Work out the finished part from the listing and answer in its coordinate system (mm). Round coordinates to 2 decimals unless told otherwise and drop trailing zeros. Order: outer loops, then holes, each group sorted by start corner. A loop starts at its lowest first (then second) coordinate and runs counter-clockwise, first axis right, second up. Notation, with made-up numbers: (78.25, -34) - (87.25, -34) arc R12 cw to (87.25, -18) - close; hole circle Ø2 at (1.25, 56.5). An arc over 180 degrees is marked (long way). Answer in a Markdown table with one row per item.
from build123d import *

# Parameters (mm, degrees)
SKETCH1_R           = 1.75
SKETCH1_R_2         = 1
BOSS_EXTRUDE1_DEPTH = 2
SKETCH3_R           = 1.75
SKETCH3_W           = 40
SKETCH3_H           = 10
CUT_EXTRUDE2_DEPTH  = 10
FILLET1_R           = 2
FILLET2_R           = 5
FILLET3_R           = 10
SKETCH4_R           = 1.5
CUT_EXTRUDE3_DEPTH  = 10


with BuildPart() as part:
    # Sketch1 → Boss-Extrude1 (new body)
    with BuildSketch(Plane(origin=(0, 0, 0), x_dir=(1, 0, 0), z_dir=(0, 1, 0))):
        Polygon((-90, 32.535953793), (-90, -32.464046207), (90, -32.464046207), (90, 32.535953793), (50, 32.535953793), (50, 72.535953793), (-50, 72.535953793), (-50, 32.535953793), align=None)
        with Locations((-85, -27.535953793)):
            Circle(SKETCH1_R, mode=Mode.SUBTRACT)
        with Locations((85, -27.535953793)):
            Circle(SKETCH1_R, mode=Mode.SUBTRACT)
        with Locations((-30, -27.535953793)):
            Circle(SKETCH1_R, mode=Mode.SUBTRACT)
        with Locations((30, -27.535953793)):
            Circle(SKETCH1_R, mode=Mode.SUBTRACT)
        with Locations((-67, 17.464046207)):
            Circle(SKETCH1_R, mode=Mode.SUBTRACT)
        with Locations((67, 17.464046207)):
            Circle(SKETCH1_R, mode=Mode.SUBTRACT)
        with Locations((-47, 69.535953793)):
            Circle(SKETCH1_R_2, mode=Mode.SUBTRACT)
        with Locations((-47, 25.035953793)):
            Circle(SKETCH1_R_2, mode=Mode.SUBTRACT)
        with Locations((47, 25.035953793)):
            Circle(SKETCH1_R_2, mode=Mode.SUBTRACT)
        with Locations((47, 69.535953793)):
            Circle(SKETCH1_R_2, mode=Mode.SUBTRACT)
    extrude(amount=BOSS_EXTRUDE1_DEPTH)

    # Sketch3 → Cut-Extrude2 (cut)
    with BuildSketch(Plane(origin=(0, 2, 0), x_dir=(1, 0, 0), z_dir=(0, 1, 0))):
        with Locations((-43, 62.464046207)):
            Circle(SKETCH3_R)
        with Locations((43, 62.464046207)):
            Circle(SKETCH3_R)
        Polygon((2.5, 48.535953793), (42.5, 48.535953793), (42.5, 46.535953793), (38, 46.535953793), (38, 6.535953793), (25, 6.535953793), (25, -13.464046207), (-25, -13.464046207), (-25, 6.535953793), (-38, 6.535953793), (-38, 46.535953793), (-42.5, 46.535953793), (-42.5, 48.535953793), (-2.5, 48.535953793), (-2.5, 53.535953793), (2.5, 53.535953793), align=None)
        with Locations((70, 27.535953793)):
            Rectangle(SKETCH3_W, SKETCH3_H)
        with Locations((-70, 27.535953793)):
            Rectangle(SKETCH3_W, SKETCH3_H)
    extrude(amount=-CUT_EXTRUDE2_DEPTH, mode=Mode.SUBTRACT)

    # Fillet1
    fillet1_edges = [part.edges().sort_by_distance(p)[0] for p in [
        (-50, 1, -72.535953793),
        (50, 1, -72.535953793),
    ]]
    fillet(fillet1_edges, radius=FILLET1_R)

    # Fillet2
    fillet2_edges = [part.edges().sort_by_distance(p)[0] for p in [
        (90, 1, -22.535953793),
        (25, 1, -6.535953793),
        (-25, 1, -6.535953793),
        (90, 1, 32.464046207),
        (-90, 1, 32.464046207),
        (-90, 1, -22.535953793),
    ]]
    fillet(fillet2_edges, radius=FILLET2_R)

    # Fillet3
    fillet3_edges = [part.edges().sort_by_distance(p)[0] for p in [
        (50, 1, -22.535953793),
        (-50, 1, -22.535953793),
    ]]
    fillet(fillet3_edges, radius=FILLET3_R)

    # Sketch4 → Cut-Extrude3 (cut)
    with BuildSketch(Plane(origin=(0, 2, 0), x_dir=(1, 0, 0), z_dir=(0, 1, 0))):
        with Locations((-82, 10.535953793)):
            Circle(SKETCH4_R)
        with Locations((-82, -4.464046207)):
            Circle(SKETCH4_R)
        with Locations((82, 10.535953793)):
            Circle(SKETCH4_R)
        with Locations((82, -4.464046207)):
            Circle(SKETCH4_R)
    extrude(amount=-CUT_EXTRUDE3_DEPTH, mode=Mode.SUBTRACT)


solid = part.part
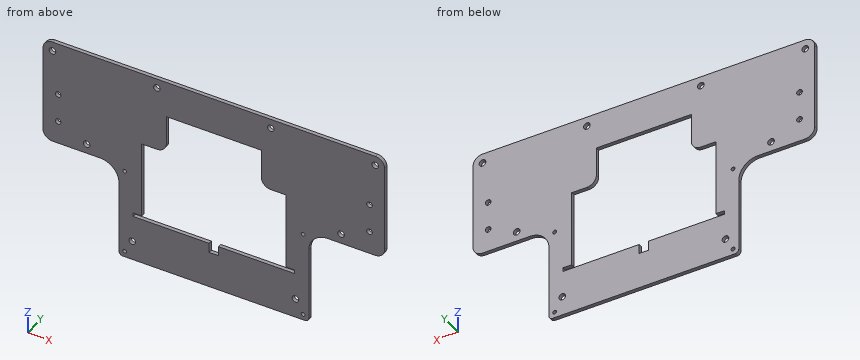
1) Find section A-A, the plane x = 18.5. Give the vertices of the cut face in (y, z).
Filled in:
| item | result |
|---|---|
| outline | (0, -72.54) - (2, -72.54) - (2, -48.54) - (0, -48.54) - close; (0, 13.46) - (2, 13.46) - (2, 32.46) - (0, 32.46) - close |
2) This flat-tipped pin is pushed along its axis until it touches: pin 1 (0.6 mm diameter, centred on y = 0.5, z = -43.5, fed in from -X). Where does it stop, or does it pass through?
Filled in:
| item | result |
|---|---|
| pin 1 | stops at x = -50 |
3) Find section C-C, the plane y = 1.7. Give the number of separate pieces and of enclosed holes in the cut face, then the cut area to 3 significant figures.
Filled in:
| item | result |
|---|---|
| separate pieces | 1 |
| enclosed holes | 17 |
| area | 10,600 mm^2 |
4) Find section D-D, the plane x = 63. Give the vertices of the cut face in (y, z).
Filled in:
| item | result |
|---|---|
| outline | (0, -22.54) - (2, -22.54) - (2, 32.46) - (0, 32.46) - close |
5) Find the intervals of material crossed by probe 1 along Z at (x, y) = (30, 0.5); probe 2 along X at (y, z) = (0.7, -10.5); probe 3 along Z at (x, y) = (47, 0.6), in increasing order. Write a range as from..to.
Filled in:
| item | result |
|---|---|
| probe 1 | z = -72.54..-48.54, -6.54..25.79, 29.29..32.46 |
| probe 2 | x = -90..-83.5, -80.5..-38, 38..80.5, 83.5..90 |
| probe 3 | z = -72.54..-70.54, -68.54..-26.04, -24.04..32.46 |
6) Find section B-B, the plane z = 10.5. Give the vertices of the cut face in (x, y), then the cut area to 3 significant figures.
Filled in:
| item | result |
|---|---|
| outline | (-90, 0) - (-25, 0) - (-25, 2) - (-90, 2) - close; (25, 0) - (90, 0) - (90, 2) - (25, 2) - close |
| area | 260 mm^2 |
